Source: CAD feature listing. Evaluate the final solid. Frame: model axes, mm. Face numbers are marked on the shaded views. A direction names the side the tool comes from. Coordinates: 2 decimals unless noted, no trailing zeros. Order: outer loops, then holes, each group sorted by start corner. A loop starts at its lowest first (then second) coordinate and runs counter-clockwise, first axis right, second up. Notation, with made-up numbers: (-24.5, 27) - (14.5, 27) arc R19 ccw to (14.5, 31) - close; hole circle Ø9 at (59, -20.5). An arc over 180 degrees is marked (long way). One line per question, with ' | ' between items. Start each with the question number.
(1) Section C-C (x = -3). Return the cut outline in (y, z), then the cut area to 3 significant figures.
(2) Line query: line 1 along X through (y, z) = (8.5, -21.5); line 2 along Z through (x, y) = (2, 1.85); line 3 along Z through (x, y) = (2, 6.4). Output: solid intervals per line, ascending.
(3) Section B-B (z = 4). Return the cut outline in (x, y), then the cut area to 3 significant figures.
(4) Section A-A (y = 7.5). Return the cut outline in (x, z).
(5) Draft query along X for the marked faces 6, 7 and 8. Return one class per face: +X half, -X half, draft (parallel to the pull), parting line (faces both ways), or undercut.
(6) Access query for the marked faces 1, 2, 3, 4 and 5. Directions: +Z, -Z, +X, -X, +Y, -Y. A direction counts if a zero-diameter tool reaches every point of the face in a straight line with its end or side. Return the directions, or none.
(7) Contact query for flat-ended pins moving along their axis: P1, Ø9, axis at x = 0, z = 0, coming from the +Y side; P2, Ø5, axis at x = -9.9, z = -9.9, coming from the -Y side; P3, Ø3, axis at x = -2.5, y = 6.5, coming from the -Z side; P4, Ø23, axis at x = -3.5, z = -2.5, coming from the +Y side. Output: stop coordinate, or through.
(8) Section D-D (z = -21.5). Return the cut outline in (x, y), then the cut area to 3 significant figures.
from build123d import *

# Parameters (mm, degrees)
SKETCH1_R           = 30
SKETCH1_R_2         = 5
BOSS_EXTRUDE1_DEPTH = 4
SKETCH4_R           = 10.5
SKETCH4_R_2         = 8
BOSS_EXTRUDE2_DEPTH = 5
SKETCH6_R           = 1.5
CUT_EXTRUDE3_DEPTH  = 5
SKETCH7_R           = 1.5
BOSS_EXTRUDE3_DEPTH = 6
SKETCH8_R           = 1.5
CUT_EXTRUDE4_DEPTH  = 5


with BuildPart() as part:
    # Sketch1 → Boss-Extrude1 (new body)
    with BuildSketch(Plane(origin=(0, 0, 0), x_dir=(1, 0, 0), z_dir=(0, 1, 0))):
        Circle(SKETCH1_R)
        Circle(SKETCH1_R_2, mode=Mode.SUBTRACT)
    extrude(amount=BOSS_EXTRUDE1_DEPTH)

    # Sketch4 → Boss-Extrude2 (add)
    with BuildSketch(Plane(origin=(0, 4, 0), x_dir=(1, 0, 0), z_dir=(0, 1, 0))):
        Circle(SKETCH4_R)
        Circle(SKETCH4_R_2, mode=Mode.SUBTRACT)
    extrude(amount=BOSS_EXTRUDE2_DEPTH)

    # Sketch6 → Cut-Extrude3 (cut, through all)
    with BuildSketch(Plane(origin=(0, 4, 0), x_dir=(1, 0, 0), z_dir=(0, 1, 0))):
        with Locations((-7.5, 21.5)):
            Circle(SKETCH6_R)
        with Locations((2, 21.5)):
            Circle(SKETCH6_R)
    extrude(amount=-CUT_EXTRUDE3_DEPTH, mode=Mode.SUBTRACT)

    # Sketch7 → Boss-Extrude3 (add)
    with BuildSketch(Plane(origin=(0, 4, 0), x_dir=(1, 0, 0), z_dir=(0, 1, 0))):
        with BuildLine():
            Line((2, 25.5), (-7.5, 25.5))
            ThreePointArc((-7.5, 25.5), (-11.5, 21.5), (-7.5, 17.5))
            Line((-7.5, 17.5), (2, 17.5))
            ThreePointArc((2, 17.5), (6, 21.5), (2, 25.5))
        make_face()
        with Locations((-7.5, 21.5)):
            Circle(SKETCH7_R, mode=Mode.SUBTRACT)
        with Locations((2, 21.5)):
            Circle(SKETCH7_R, mode=Mode.SUBTRACT)
    extrude(amount=BOSS_EXTRUDE3_DEPTH)

    # Sketch8 → Cut-Extrude4 (cut, through all)
    with BuildSketch(Plane(origin=(0, 4, 0), x_dir=(1, 0, 0), z_dir=(0, 1, 0))):
        with Locations((-9.899494937, 9.899494937)):
            Circle(SKETCH8_R)
        with Locations((9.899494937, 9.899494937)):
            Circle(SKETCH8_R)
        with Locations((9.899494937, -9.899494937)):
            Circle(SKETCH8_R)
        with Locations((-9.899494937, -9.899494937)):
            Circle(SKETCH8_R)
    extrude(amount=-CUT_EXTRUDE4_DEPTH, mode=Mode.SUBTRACT)


solid = part.part
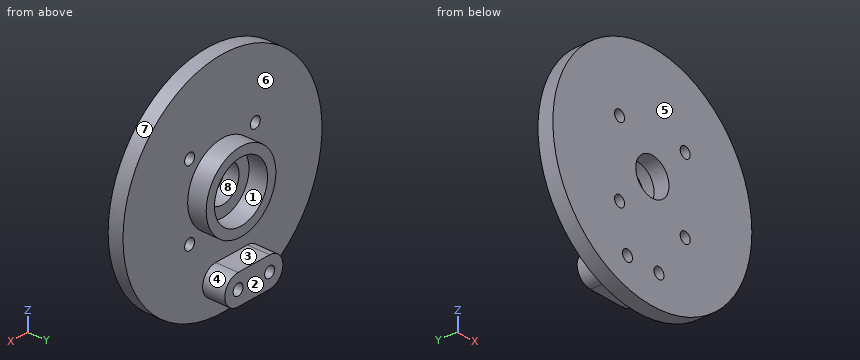
Response values:
1) outline: (0, -29.85) - (4, -29.85) - (4, -25.5) - (10, -25.5) - (10, -17.5) - (4, -17.5) - (4, -10.06) - (9, -10.06) - (9, -7.42) - (4, -7.42) - (4, -4) - (0, -4) - close; (0, 4) - (4, 4) - (4, 7.42) - (9, 7.42) - (9, 10.06) - (4, 10.06) - (4, 29.85) - (0, 29.85) - close | area: 281 mm²
2) line 1: x = -11.5 to -9, -6 to 0.5, 3.5 to 6 | line 2: z = -29.93 to -23, -20 to -4.58, 4.58 to 29.93 | line 3: z = -25.5 to -23, -20 to -17.5, -10.31 to -7.75, 7.75 to 10.31
3) outline: (-29.73, 0) - (-3, 0) - (-3, 4) - (-6.93, 4) - (-6.93, 9) - (-9.71, 9) - (-9.71, 4) - (-29.73, 4) - close; (3, 0) - (29.73, 0) - (29.73, 4) - (9.71, 4) - (9.71, 9) - (6.93, 9) - (6.93, 4) - (3, 4) - close | area: 242 mm²
4) outline: circle Ø21 at (0, 0); (-7.5, -25.5) - (2, -25.5) arc R4 ccw to (2, -17.5) - (-7.5, -17.5) arc R4 ccw to start; hole circle Ø3 at (-7.5, -21.5); hole circle Ø16 at (0, 0); hole circle Ø3 at (2, -21.5)
5) face 6: draft | face 7: parting line | face 8: undercut
6) face 1: +Y | face 2: +Z, -Z, +X, -X, +Y | face 3: +X, -X, +Y | face 4: +X, +Y | face 5: +Z, -Z, +X, -X, -Y
7) P1: passes through | P2: stops at y = 0 | P3: stops at z = -25.5 | P4: stops at y = 9
8) outline: (-20.92, 0) - (-9, 0) - (-9, 10) - (-11.5, 10) - (-11.5, 4) - (-20.92, 4) - close; (-6, 0) - (0.5, 0) - (0.5, 10) - (-6, 10) - close; (3.5, 0) - (20.92, 0) - (20.92, 4) - (6, 4) - (6, 10) - (3.5, 10) - close | area: 212 mm²
